Check sheet for the modelled part. Datum: model origin and axes. Units: mm. Face numbers are marked on the shaded views. Give positions to 0.01 mm unless a question says otherwise; leave off trailing zeros. Loops run counter-clockwise (first coordinate to the right, second up) from the corner with the lowest first, then second, coordinate; pieces in that order, holes last. Notation, with made-up numbers: M 41,11.25 L 85,11.25 A17 cw 85,38.25 Z; hole C 39.25,-21 d11. An arc over 180 degrees is marked long. One line per question, with ' | ' between items. Start each with the question number.
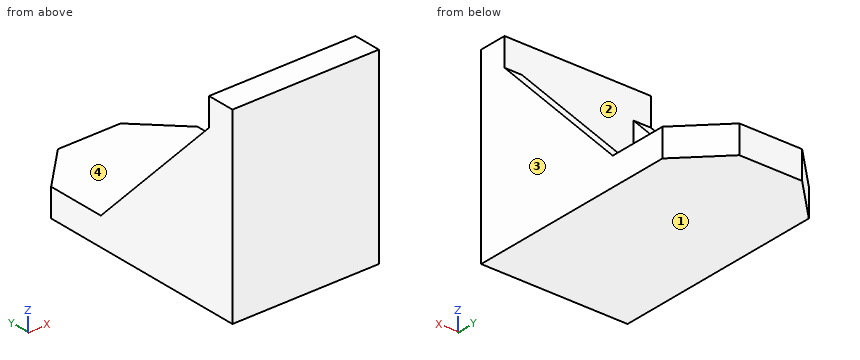
from build123d import *

# Parameters (mm, degrees)
BOSS_EXTRUDE1_DEPTH = 8
SKETCH2_W           = 42
SKETCH2_H           = 8
BOSS_EXTRUDE2_DEPTH = 46
BOSS_EXTRUDE3_DEPTH = 5


with BuildPart() as part:
    # Sketch1 → Boss-Extrude1 (new body)
    with BuildSketch(Plane.XY):
        Polygon((0, 0), (0, 62), (12, 74), (30, 74), (42, 62), (42, 0), align=None)
    extrude(amount=BOSS_EXTRUDE1_DEPTH)

    # Sketch2 → Boss-Extrude2 (add)
    with BuildSketch(Plane.XY.offset(8)):
        with Locations((21, 4)):
            Rectangle(SKETCH2_W, SKETCH2_H)
    extrude(amount=BOSS_EXTRUDE2_DEPTH)

    # Sketch3 → Boss-Extrude3 (add)
    with BuildSketch(Plane(origin=(42, 0, 0), x_dir=(0, 0, -1), z_dir=(1, 0, 0))):
        Polygon((-8, 8), (-8, 45), (-46, 8), align=None)
    extrude(amount=-BOSS_EXTRUDE3_DEPTH)

    # Mirror1: part across plane


with BuildPart() as part_1:
    add(part.part)
    add(part.part.mirror(Plane(origin=(21, 0, 0), x_dir=(0, 0, 1), z_dir=(1, 0, 0))))


solid = part_1.part
Q1. Cross-section at C-C (y = 27). Record the cut outline in (x, z), and give its area (3 significant figures).
Q2. Cross-section at A-A (z = 27). Record the cut outline in (x, y).
Q3. Cross-section at B-B (x = 4). Record the cut outline in (y, z).
Q4. Depth check by flat-ended pin: P1, Ø8, axis at x = 32, z = 41.5, coming from the +Y side; P2, Ø10, axis at x = 22, y = 37.5, coming from the -Z side; P3, Ø1, axis at x = 16, y = 34, coming from the +Z side. Enter the tip coordinate at first touch or a pass-through.
Q5. Cross-section at D-D (x = 32). Record the cut outline in (y, z), and give its area (3 significant figures).
Q6. Material ranges on probe 1 along X at (y, z) = (35.5, 15); probe 2 along Z at (x, y) = (18, 27), recorded low to high. Write a range as from..to.
Q7. Draft check along X on the marked faces 1, 2, 3 and 4. Enter one of: released by +X, released by -X, zero draft, split by the parting line, or undercut.
Solved:
1) outline: M 0,0 L 42,0 L 42,26.49 L 37,26.49 L 37,8 L 5,8 L 5,26.49 L 0,26.49 Z | area: 521 mm²
2) outline: M 0,0 L 42,0 L 42,26.5 L 37,26.5 L 37,8 L 5,8 L 5,26.5 L 0,26.5 Z
3) outline: M 0,0 L 66,0 L 66,8 L 45,8 L 8,46 L 8,54 L 0,54 Z
4) P1: stops at y = 8 | P2: stops at z = 0 | P3: stops at z = 8
5) outline: M 0,0 L 72,0 L 72,8 L 8,8 L 8,54 L 0,54 Z | area: 944 mm²
6) probe 1: x = 0..5, 37..42 | probe 2: z = 0..8
7) face 1: zero draft | face 2: undercut | face 3: released by +X | face 4: undercut
